```python
from build123d import *

# Parameters (mm, degrees)
F1_DEPTH = 12.7
F2_W     = 59.3439098448
F2_H     = 33.9378900826
F3_DEPTH = 12.7
F4_W     = 39.1593687236
F4_H     = 35.0508086056
F5_DEPTH = 12.7


with BuildPart() as f1:
    # F0 (on Front) → F1 (new body)
    with BuildSketch(Plane.XZ):
        with BuildLine():
            Line((-36.9714461267, 53.8455955684), (-52.897606045, 53.8455955684))
            Line((-52.897606045, 53.8455955684), (-52.897606045, -84.0487536043))
            Line((-52.897606045, -84.0487536043), (6.4463037997, -84.0487536043))
            Line((6.4463037997, -84.0487536043), (6.4463037997, 53.8455955684))
            Line((6.4463037997, 53.8455955684), (-8.5318721831, 53.8455955684))
            Line((-8.5318721831, 53.8455955684), (-8.5318721831, 25.0268243253))
            ThreePointArc((-8.5318721831, 25.0268243253), (-22.7516591549, 10.8070373535), (-36.9714461267, 25.0268243253))
            Line((-36.9714461267, 25.0268243253), (-36.9714461267, 53.8455955684))
        make_face()
    extrude(amount=F1_DEPTH)

    # F2 (on face) → F3 (join)
    with BuildSketch(Plane(origin=(0, 0, -84.0487536043), x_dir=(1, 0, 0), z_dir=(0, 0, -1))):
        with Locations((-23.2256511226, 16.9689450413)):
            Rectangle(F2_W, F2_H)
        with BuildLine():
            Line((-52.897606045, 33.9378900826), (6.4463037997, 33.9378900826))
            ThreePointArc((6.4463037997, 33.9378900826), (-23.2256511226, 63.609845005), (-52.897606045, 33.9378900826))
        make_face()
    extrude(amount=F3_DEPTH)

    # F4 (on face) → F5 (cut)
    with BuildSketch(Plane.YZ.offset(6.4463037997)):
        with Locations((-19.5796843618, -79.2233493015)):
            Rectangle(F4_W, F4_H)
    extrude(amount=-F5_DEPTH, mode=Mode.SUBTRACT)


solid = f1.part
```
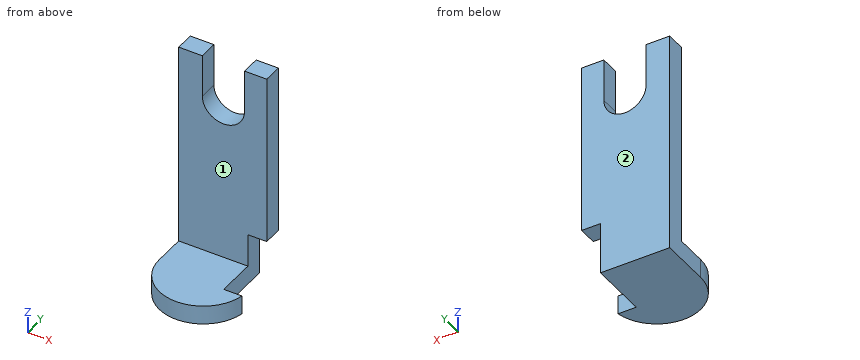
The listing builds one solid part. Answer for the finished solid, in the listing's coordinates (mm). Face numbers are marked on the shaded views. A direction names the side the tool comes from. Give positions to 0.01 mm unless a question says otherwise; leave off trailing zeros. Write each loop counter-clockwise with the first axis right and the second up, starting at its lowest first coordinate (ties: lowest second). Pieces come first, ordered by that corner, then holes. Notation, with made-up numbers: M 23.25,-38 L 66.25,-38 A29 ccw 66.25,-14 Z; hole C -6.5,88 d4. An arc over 180 degrees is marked long. Write each question's results on one line, items separated by ' | '.
Q1. Flat-ended cylindrical pins translate along their axes: P1, Ø10, axis at x = -31, z = -17, coming from the -Y side; P2, Ø1, axis at x = -43, y = -45, coming from the +Z side; P3, Ø4, axis at x = 0, y = -5, coming from the -Z side. Find the tip coordinate at first contact, or state that the pin passes through.
Output values:
P1: y = -12.7 | P2: z = -84.05 | P3: z = -61.7
Q2. A tool of negligible diameter and unlimited length cuts with its end or side. For the marked faces 1 and 2, from which of +Z, -Z, +X, -X, +Y, -Y can it reach the whole face along a straight path? Write none if from no direction.
Output values:
face 1: +Z, +X, -X, -Y | face 2: +Z, -Z, +X, -X, +Y
Q3. Section D-D, the plane z = -79 is taken. Write down the section's boundary in (x, y), then the cut area to 3 significant figures.
Output values:
outline: M -52.9,-12.7 L -6.25,-12.7 L -6.25,0 L -52.9,0 Z | area: 592 mm2
Q4. Section A-A, the plane z = 35 is taken. Write down the section's boundary in (x, y).
Output values:
outline: M -52.9,-12.7 L -36.97,-12.7 L -36.97,0 L -52.9,0 Z; M -8.53,-12.7 L 6.45,-12.7 L 6.45,0 L -8.53,0 Z
Q5. Section C-C, the plane y = -20.5 is taken. Write down the section's boundary in (x, z), then the cut area to 3 significant figures.
Output values:
outline: M -52.9,-96.75 L -6.25,-96.75 L -6.25,-84.05 L -52.9,-84.05 Z | area: 592 mm2
Q6. Section B-B, the plane x = -0.5 is taken. Write down the section's boundary in (y, z), then the cut area to 3 significant figures.
Output values:
outline: M -53.02,-96.75 L -39.16,-96.75 L -39.16,-84.05 L -53.02,-84.05 Z; M -12.7,-61.7 L 0,-61.7 L 0,53.85 L -12.7,53.85 Z | area: 1,640 mm2
Q7. Consider L1, parallel to Z at x = -34, y = -35; L2, parallel to Y at x = -28, z = -72.5; L3, parallel to X at y = -7, z = 14.5. Determine where each line is inside the solid, lowest interval first. Write a range as from..to.
Output values:
L1: -96.75..-84.05 | L2: -12.7..0 | L3: -52.9..-32.31, -13.19..6.45
